Design review of the part built by this model. Coordinates are the model's own, in mm. Face numbers are marked on the shaded views. A direction names the side the tool comes from. Give positions to 0.01 mm unless a question says otherwise; leave off trailing zeros. Order: outer loops, then holes, each group sorted by start corner. A loop starts at its lowest first (then second) coordinate and runs counter-clockwise, first axis right, second up. Notation, with made-up numbers: (67.5, -40) -> (115.5, -40) arc R24 ccw to (115.5, -26) -> close; hole circle Ø5 at (-30, -30). An arc over 180 degrees is marked (long way). One line per item, written item: value. Start each with the question number.
1) Tool access review of the marked faces 1 and 2: name each direction out of +Z, -Z, +X, -X, +Y, -Y from which nothing blocks a thin tool from reaching the whole face with its end or side.
2) Consider section C-C (y = 168). State the section outline as (x, z) points.
3) For pin 1 (1 mm diameter, centred on x = 2.5, y = 320.5, fed in from +Z); pin 2 (10 mm diameter, centred on x = -1.5, y = 291, fed in from -Z); pin 3 (8 mm diameter, centred on y = 142, z = 2, fed in from -X), all flat-tipped, find the tip position at first contact; note any pin that passes through.
4) Wall thickness on line 1 along Y through (x, z) = (7.5, 2.5); line 2 along Z through (x, y) = (0.25, 154): over which ranges is each line inside the solid? List them lowest first. Write a range as from..to.
5) Consider section A-A (z = 0). State the section outline as (x, y) points (3 decimals).
6) Consider section B-B (x = 0). State the section outline as (y, z) points (3 decimals).
Autodesk Inventor part; units mm, degrees
ref_plane "YZ Plane" through (0, 0, 0) normal (1, 0, 0) x (0, 1, 0)
ref_plane "XZ Plane" through (0, 0, 0) normal (0, 1, 0) x (-1, 0, 0)
ref_plane "XY Plane" through (0, 0, 0) normal (0, 0, 1) x (1, 0, 0)
sketch "Sketch1" plane through (0, 0, 0) normal (0, 1, 0) x (-1, 0, 0)
  circle A0 centre (0, 0) radius 9.525
  dimension "d0" = 19.05
extrude "Extrusion1" add sketch "Sketch1" along normal blind 2.54
sketch "Sketch2" plane through (0, 2.54, 0) normal (0, 1, 0) x (1, 0, 0)
  circle A0 centre (0, 0) radius 9.525
  circle A1 centre (0, 0) radius 6.35
  dimension "d3" = 12.7
extrude "Extrusion2" add sketch "Sketch2" along normal blind 177.8 contours A1
mirror "Mirror1" about plane through (0, 180.34, 0) normal (0, 1, 0) of "Extrusion1"
mirror "Mirror2" about plane through (0, 180.34, 0) normal (0, 1, 0) of "Extrusion2"
properties part number "pole 1"
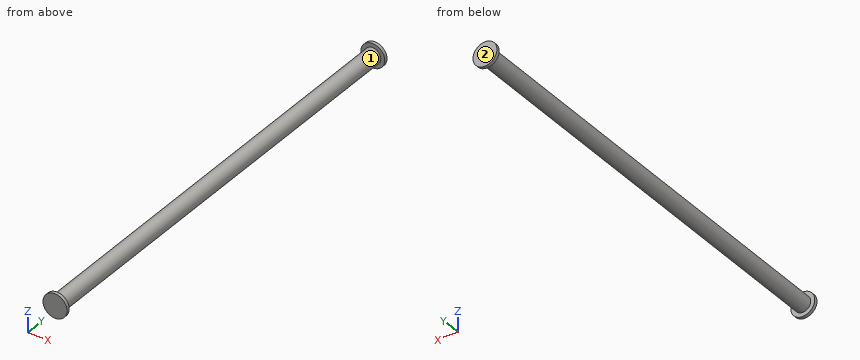
Checked values:
1. face 1: none
1. face 2: +Z, -Z, +X, -X, +Y
2. outline: circle Ø12.7 at (0, 0)
3. pin 1: stops at z = 6.03
3. pin 2: stops at z = -6.35
3. pin 3: stops at x = -6.35
4. line 1: y = 0..2.54, 358.14..360.68
4. line 2: z = -6.35..6.35
5. outline: (-9.525, 0) -> (9.525, 0) -> (9.525, 2.54) -> (6.35, 2.54) -> (6.35, 358.14) -> (9.525, 358.14) -> (9.525, 360.68) -> (-9.525, 360.68) -> (-9.525, 358.14) -> (-6.35, 358.14) -> (-6.35, 2.54) -> (-9.525, 2.54) -> close
6. outline: (0, -9.525) -> (2.54, -9.525) -> (2.54, -6.35) -> (358.14, -6.35) -> (358.14, -9.525) -> (360.68, -9.525) -> (360.68, 9.525) -> (358.14, 9.525) -> (358.14, 6.35) -> (2.54, 6.35) -> (2.54, 9.525) -> (0, 9.525) -> close
